Input: dimensioned drawing with shaded views. Units: mm. Origin: part minimum x, y, z. A direction names the side the tool comes from. Round coordinates to 2 decimals unless told otherwise and drop trailing zeros. Write each loop counter-clockwise with the first axis right and the second up, starting at its lowest first coordinate (ties: lowest second). Pieces come first, ordered by that corner, then holes. Notation, with made-up numbers: (21, -30) - (50, -30) arc R25 cw to (50, -4) - close; hole circle Ø6 at (7, 14.25). An arc over 180 degrees is marked (long way). Use one line per item in the form item = value.
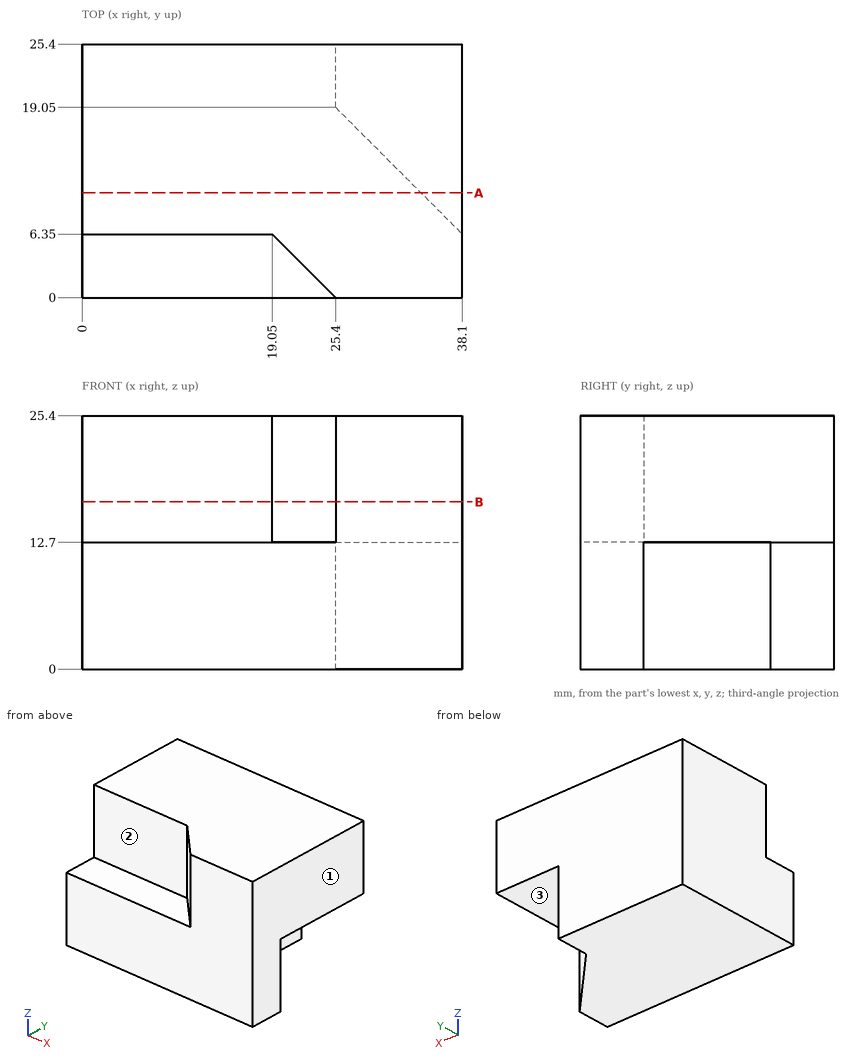
(1) First-contact query: pin 1 Ø6.5 at (x, z) = (11, 17) entering from -Y; pin 2 Ø3 at (x, y) = (12, 4) entering from +Z; pin 3 Ø3 at (y, z) = (21.5, 8.5) entering from +X. Flat tips, straight axial feed; report the tip coordinate or a pass-through.
Derived:
pin_1 = 6.35
pin_2 = 12.7
pin_3 = 25.4
(2) Cut plane B-B on z = 16.75. Output: boundary loops of the cut face in (x, y), then the cut area to 3 significant figures.
Derived:
outline = (0, 6.35) - (19.05, 6.35) - (25.4, 0) - (38.1, 0) - (38.1, 25.4) - (0, 25.4) - close
area = 827 mm^2
(3) Material intervals for L1, parallel to X at y = 20.25, z = 10; L2, parallel to Z at x = 9.5, y = 2.5; L3, parallel to Y at x = 6.5, z = 21.75, sorted ascending.
Derived:
L1 = 0 to 25.4
L2 = 0 to 12.7
L3 = 6.35 to 25.4
(4) Access query for the marked faces 1, 2 and 3. Directions: +Z, -Z, +X, -X, +Y, -Y. A direction counts if a zero-diameter tool reaches every point of the face in a straight line with its end or side. Return the directions, or none.
Derived:
face_1 = +Z, -Z, +X, +Y, -Y
face_2 = +Z, -X, -Y
face_3 = -Z, +X, +Y
(5) Cut plane A-A on y = 10.5. Output: boundary loops of the cut face in (x, z).
Derived:
outline = (0, 0) - (33.95, 0) - (33.95, 12.7) - (38.1, 12.7) - (38.1, 25.4) - (0, 25.4) - close
